Read the model definition and answer for the solid it produces. Units are mm, in the model's axes. Face numbers are marked on the shaded views. A direction names the side the tool comes from. Coordinates: 2 decimals unless noted, no trailing zeros. Loops run counter-clockwise (first coordinate to the right, second up) from the corner with the lowest first, then second, coordinate; pieces in that order, holes last. Notation, with made-up numbers: (4.5, 48.5) -> (55.5, 48.5) arc R20 cw to (55.5, 64.5) -> close; hole circle Ø7 at (-28, -5). An arc over 180 degrees is marked (long way). Answer as a JSON object with one key per item and string values. Group by question number.
Q1. Determine the mould class of the marked faces 3, 4 and 5 for opening direction Z: released by +Z, released by -Z, zero draft, split by the parting line, or undercut.
Q2. The part is cut by section D-D on y = 5.5. Write down the section's boundary in (x, z), and give its area (3 significant figures).
Q3. This flat-tipped pin is pushed along its axis until it touches: P1, Ø2, axis at x = -0.5, z = 0, coming from the +Y side. Where does it stop, or does it pass through?
Q4. Straight lines are drawn through the part: line 1 along X through (y, z) = (12.65, 0); line 2 along Y through (x, z) = (0.95, 0.55); line 3 along Y through (x, z) = (-1.85, 1.9). For each, find the intervals that lie inside material, in ascending order. Write a range as [from, to].
Q5. The part is cut by section A-A on z = 0. Write down the section's boundary in (x, y).
Q6. For the marked faces 1 and 2, determine the directions among +Z, -Z, +X, -X, +Y, -Y from which every point of the face is accessible in a straight line to the end or side of a thin tool.
Q7. The part is cut by section C-C on x = 0. Write down the section's boundary in (y, z), and give its area (3 significant figures).
Q8. The part is cut by section B-B on y = 12.5. Write down the section's boundary in (x, z).
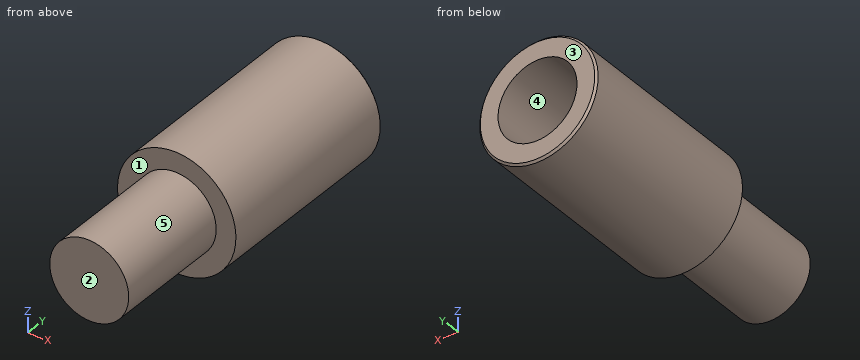
from build123d import *

# Parameters (mm, degrees)
SKETCH1_R           = 2
BOSS_EXTRUDE1_DEPTH = 6
SKETCH2_R           = 3
BOSS_EXTRUDE2_DEPTH = 10
CUT_EXTRUDE1_START  = -6
SKETCH3_R           = 2
CUT_EXTRUDE1_DEPTH  = 6
CHAMFER1_SIZE       = 0.1


with BuildPart() as part:
    # Sketch1 → Boss-Extrude1 (new body)
    with BuildSketch(Plane(origin=(0, 0, 0), x_dir=(1, 0, 0), z_dir=(0, 1, 0))):
        with Locations(Location((0, 0, 0), (0, 0, 270))):
            Circle(SKETCH1_R)
    extrude(amount=BOSS_EXTRUDE1_DEPTH)

    # Sketch2 → Boss-Extrude2 (add)
    with BuildSketch(Plane(origin=(0, 6, 0), x_dir=(1, 0, 0), z_dir=(0, 1, 0))):
        with Locations(Location((0, 0, 0), (0, 0, 270))):
            Circle(SKETCH2_R)
    extrude(amount=BOSS_EXTRUDE2_DEPTH)

    # Sketch3 → Cut-Extrude1 (cut)
    with BuildSketch(Plane(origin=(0, 16, 0), x_dir=(1, 0, 0), z_dir=(0, 1, 0)).offset(CUT_EXTRUDE1_START)):
        with Locations(Location((0, 0, 0), (0, 0, 270))):
            Circle(SKETCH3_R)
    extrude(amount=CUT_EXTRUDE1_DEPTH, mode=Mode.SUBTRACT)

    # Chamfer1
    chamfer1_edges = [part.edges().sort_by_distance(p)[0] for p in [
        (0, 16, -3),
    ]]
    chamfer(chamfer1_edges, length=CHAMFER1_SIZE)


solid = part.part
Final values:
{
 "1": {"face 3": "zero draft", "face 4": "undercut", "face 5": "split by the parting line"},
 "2": {"outline": "circle Ø4 at (0, 0)", "area": "12.6 mm2"},
 "3": {"P1": "stops at y = 10"},
 "4": {"line 1": "x = [-3, -2], [2, 3]", "line 2": "y = [0, 10]", "line 3": "y = [6, 16]"},
 "5": {"outline": "(-3, 6) -> (-2, 6) -> (-2, 0) -> (2, 0) -> (2, 6) -> (3, 6) -> (3, 15.9) -> (2.9, 16) -> (2, 16) -> (2, 10) -> (-2, 10) -> (-2, 16) -> (-2.9, 16) -> (-3, 15.9) -> close"},
 "6": {"face 1": "-Y", "face 2": "+Z, -Z, +X, -X, -Y"},
 "7": {"outline": "(0, -2) -> (6, -2) -> (6, -3) -> (15.9, -3) -> (16, -2.9) -> (16, -2) -> (10, -2) -> (10, 2) -> (16, 2) -> (16, 2.9) -> (15.9, 3) -> (6, 3) -> (6, 2) -> (0, 2) -> close", "area": "60.0 mm2"},
 "8": {"outline": "circle Ø6 at (0, 0); hole circle Ø4 at (0, 0)"}
}
